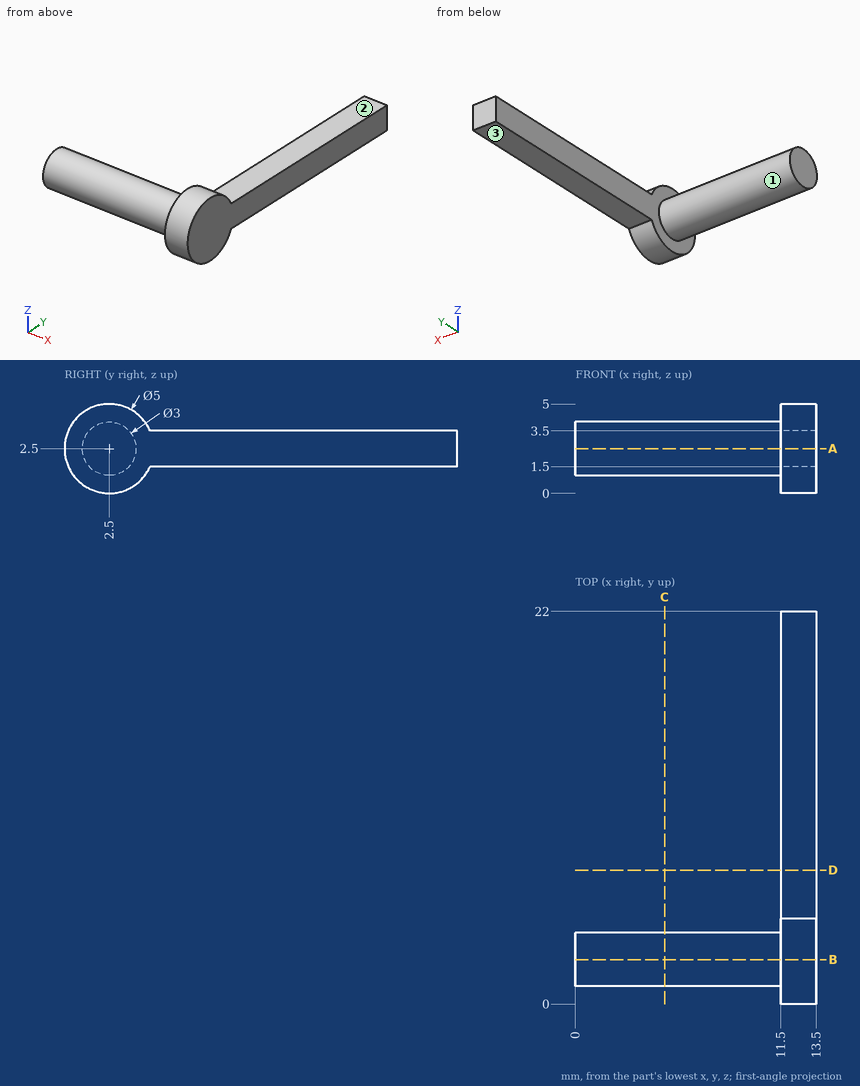
Part print with two shaded views. Sizes in mm from the minimum x, y, z corner. A direction names the side the tool comes from. Coordinates: 2 decimals unless noted, no trailing zeros. Write each loop counter-clockwise with the first axis right and the second up, starting at its lowest first coordinate (ties: lowest second). Pieces come first, ordered by that corner, then holes. Notation, with made-up numbers: (74.25, -15.5) - (132.25, -15.5) arc R7 cw to (132.25, -7.5) - close; hole circle Ø2 at (34.5, 59.5). An arc over 180 degrees is marked (long way). Put each result on its own line as item: value.
1. 3-axis set-ups, long thin cutter, end or side, ignore diameter. For the marked faces 1, 2 and 3: which of +Z, -Z, +X, -X, +Y, -Y reach the whole face in a straight line?
Final values:
face 1: -X
face 2: +Z, +X, -X, +Y
face 3: -Z, +X, -X, +Y
2. Flat gauge pins, fed straight in: pin 1 Ø3 at (y, z) = (15.5, 3) entering from -X; pin 2 Ø2 at (x, y) = (12.5, 12) entering from -Z; pin 3 Ø0.6 at (x, y) = (12.5, 17.5) entering from +Z. Where does each tip first touch, or does it go through?
Final values:
pin 1: stops at x = 11.5
pin 2: stops at z = 1.5
pin 3: stops at z = 3.5
3. Band-saw the part on B-B (y = 2.5). Write the cut outline in (x, z).
Final values:
outline: (0, 1) - (11.5, 1) - (11.5, 0) - (13.5, 0) - (13.5, 5) - (11.5, 5) - (11.5, 4) - (0, 4) - close
4. Band-saw the part on A-A (z = 2.5). Write the cut outline in (x, y), then the cut area to 3 significant figures.
Final values:
outline: (0, 1) - (11.5, 1) - (11.5, 0) - (13.5, 0) - (13.5, 22) - (11.5, 22) - (11.5, 4) - (0, 4) - close
area: 78.5 mm²
5. Probe line 1 along X through (y, z) = (9, 1.7); line 2 along Y through (x, z) = (7, 2.45); line 3 along Z through (x, y) = (12.5, 5.25). List the from-to ranges inside material, lowest first. Write a range as [from, to].
Final values:
line 1: x = [11.5, 13.5]
line 2: y = [1, 4]
line 3: z = [1.5, 3.5]
6. Band-saw the part on D-D (y = 7.5). Write the cut outline in (x, z), then the cut area to 3 significant figures.
Final values:
outline: (11.5, 1.5) - (13.5, 1.5) - (13.5, 3.5) - (11.5, 3.5) - close
area: 4.00 mm²
7. Band-saw the part on C-C (x = 5). Write the cut outline in (y, z), then the cut area to 3 significant figures.
Final values:
outline: circle Ø3 at (2.5, 2.5)
area: 7.07 mm²
